from build123d import *

# Parameters (mm, degrees)
SKETCH2_R             = 14.49115295
CUT_EXTRUDE1_DEPTH    = 51.306406252
SKETCH3_R             = 5
EXTRUDE1_DEPTH        = 10
SKETCH5_R             = 9.901602584
SKETCH5_R_2           = 7
CUT_EXTRUDE2_DEPTH    = 3
IZIM2_R               = 4
KES_EKSTR_ZYON1_DEPTH = 220
IZIM3_R               = 4
KES_EKSTR_ZYON2_DEPTH = 40


with BuildPart() as part:
    # Sketch1 → Revolve1 (revolve)
    with BuildSketch(Plane.XY, mode=Mode.PRIVATE) as revolve1_sk:
        with BuildLine():
            Line((180.080433705, 44.141017842), (173.530538009, 44.141017842))
            ThreePointArc((173.530538009, 44.141017842), (172.538729892, 41.151971535), (173.530538009, 38.162925228))
            Line((173.530538009, 38.162925228), (180.080433705, 38.162925228))
            Line((180.080433705, 38.162925228), (180.080433705, 44.141017842))
        make_face()
        with BuildLine():
            Line((186.630329401, 44.141017842), (180.080433705, 44.141017842))
            Line((180.080433705, 44.141017842), (180.080433705, 38.162925228))
            Line((180.080433705, 38.162925228), (186.630329401, 38.162925228))
            ThreePointArc((186.630329401, 38.162925228), (187.103282451, 38.934012994), (187.429565668, 39.777695512))
            ThreePointArc((187.429565668, 39.777695512), (187.540311425, 42.052840793), (186.630329401, 44.141017842))
        make_face()
        with BuildLine():
            Line((180.080433705, 38.162925228), (180.080433705, 32.650327481))
            Line((180.080433705, 32.650327481), (187.735613173, 32.650327481))
            ThreePointArc((187.735613173, 32.650327481), (187.427007794, 35.455556025), (186.630329401, 38.162925228))
            Line((186.630329401, 38.162925228), (180.080433705, 38.162925228))
        make_face()
        with BuildLine():
            ThreePointArc((173.530538009, 38.162925228), (172.733859616, 35.455556025), (172.425254237, 32.650327481))
            Line((172.425254237, 32.650327481), (180.080433705, 32.650327481))
            Line((180.080433705, 32.650327481), (180.080433705, 38.162925228))
            Line((180.080433705, 38.162925228), (173.530538009, 38.162925228))
        make_face()
        with BuildLine():
            Line((173.530538009, 44.141017842), (169.927279386, 39.777695512))
            Line((169.927279386, 39.777695512), (169.927279386, 32.650327481))
            Line((169.927279386, 32.650327481), (172.425254237, 32.650327481))
            ThreePointArc((172.425254237, 32.650327481), (172.733859616, 35.455556025), (173.530538009, 38.162925228))
            ThreePointArc((173.530538009, 38.162925228), (172.538729892, 41.151971535), (173.530538009, 44.141017842))
        make_face()
        with BuildLine():
            ThreePointArc((186.630329401, 38.162925228), (187.427007794, 35.455556025), (187.735613173, 32.650327481))
            Line((187.735613173, 32.650327481), (189.375361044, 32.650327481))
            Line((189.375361044, 32.650327481), (189.375361044, 39.777695512))
            Line((189.375361044, 39.777695512), (187.429565668, 39.777695512))
            ThreePointArc((187.429565668, 39.777695512), (187.103282451, 38.934012994), (186.630329401, 38.162925228))
        make_face()
        Polygon((189.375361044, 39.777695512), (189.375361044, 32.650327481), (191.146824361, 32.650327481), (191.146824361, 42.553378699), (189.375361044, 42.553378699), align=None)
    revolve(revolve1_sk.sketch.rotate(Axis((-32.579678715, 32.650327481, 0), (1, 0, 0)), 90), axis=Axis((-32.579678715, 32.650327481, 0), (1, 0, 0)))

    # Sketch2 → Cut-Extrude1 (cut, through all)
    with BuildSketch(Plane.ZY.offset(-169.927279386)):
        with Locations((0, 32.650327481)):
            Circle(SKETCH2_R)
        Polygon((0, 44.141017842), (-9.95122976, 38.395672661), (-9.95122976, 26.9049823), (0, 21.15963712), (9.95122976, 26.9049823), (9.95122976, 38.395672661), align=None, mode=Mode.SUBTRACT)
    extrude(amount=-CUT_EXTRUDE1_DEPTH, mode=Mode.SUBTRACT)

    # Sweep3: sweep along a curve in space
    with BuildLine() as sweep3_path:
        Line((-222.210887695, 24.006507797, -16.672116117), (-222.346014244, 12.594218126, 18.492799117))
        ThreePointArc((-202.211021283, 30.157684617, -35.625859644), (-216.32728873, 28.357408148, -30.07863194), (-222.210887695, 24.006507797, -16.672116117))
        Line((-177.748857503, 30.157684617, -35.625859644), (-202.211021283, 30.157684617, -35.625859644))
        ThreePointArc((-157.748857503, 41.483617341, -19.141829556), (-163.606721879, 33.474973508, -30.797799013), (-177.748857503, 30.157684617, -35.625859644))
        Line((-157.748857503, 48.387877179, -9.093206659), (-157.748857503, 41.483617341, -19.141829556))
        ThreePointArc((-146.882458064, 52.727054495, 0), (-154.498514664, 52.19594197, -2.719947791), (-157.748857503, 48.387877179, -9.093206659))
        Line((-33.438092351, 32.801103659, 0), (-146.882458064, 52.727054495, 0))
        ThreePointArc((-31.708124112, 32.650327481, 0), (-32.576387258, 32.688092836, 0), (-33.438092351, 32.801103659, 0))
        Line((-31.708124112, 32.650327481, 0), (169.927279386, 32.650327481, 0))
    # Sketch3 → Sweep3 (sweep)
    with BuildSketch(Plane.ZY.offset(-169.927279386)):
        with Locations((0, 32.650327481)):
            Circle(SKETCH3_R)
    sweep(path=sweep3_path.line)

    # Sketch4 → Extrude1 (add)
    with BuildSketch(Plane(origin=(-0.053050316, -4.480433927, 13.805650207), x_dir=(0.9999933205859823, -0.0011282410835596105, 0.0034764716996236633), z_dir=(-0.003654966952096285, -0.30868502023615024, 0.9511572948247765))):
        Polygon((-226.140355235, 24.796964016), (-230.374247953, 17.911654597), (-226.528341443, 10.802341238), (-218.448542214, 10.578337297), (-214.214649497, 17.463646715), (-218.060556007, 24.572960075), align=None)
    extrude(amount=-EXTRUDE1_DEPTH)

    # Sketch5 → Cut-Extrude2 (cut)
    with BuildSketch(Plane(origin=(-0.053050316, -4.480433927, 13.805650207), x_dir=(0.9999933205859823, -0.0011282410835596105, 0.0034764716996236633), z_dir=(-0.003654966952096285, -0.30868502023615024, 0.9511572948247765))):
        with Locations((-222.294448725, 17.687650656)):
            Circle(SKETCH5_R)
        with Locations(Location((-222.294448725, 17.687650656, 0), (0, 0, 270))):
            Circle(SKETCH5_R_2, mode=Mode.SUBTRACT)
    extrude(amount=-CUT_EXTRUDE2_DEPTH, mode=Mode.SUBTRACT)

    # Çizim2 → Kes-Ekstrüzyon1 (cut)
    with BuildSketch(Plane(origin=(191.146824361, 0, 0), x_dir=(0, 0, -1), z_dir=(1, 0, 0))):
        with Locations((0, 32.650327481)):
            Circle(IZIM2_R)
    extrude(amount=-KES_EKSTR_ZYON1_DEPTH, mode=Mode.SUBTRACT)

    # Çizim3 → Kes-Ekstrüzyon2 (cut)
    with BuildSketch(Plane(origin=(-0.053050316, -4.480433927, 13.805650207), x_dir=(0.9999933205859823, -0.0011282410835595914, 0.003476471699623597), z_dir=(-0.003654966952096216, -0.3086850202361507, 0.9511572948247764))):
        with Locations(Location((-222.294448725, 17.687650656, 0), (0, 0, 270))):
            Circle(IZIM3_R)
    extrude(amount=-KES_EKSTR_ZYON2_DEPTH, mode=Mode.SUBTRACT)


solid = part.part
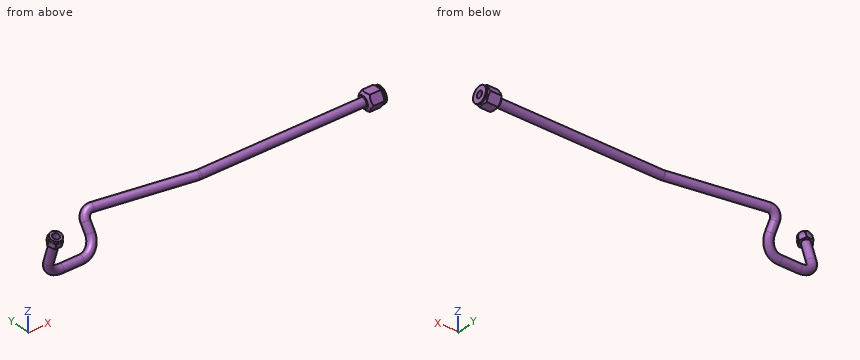
Can you work these out from the model? Positions are in its coordinate system, mm. Coordinates: 2 decimals unless noted, no trailing zeros. Order: outer loops, then holes, each group sorted by start corner. A loop starts at its lowest first (then second) coordinate and runs counter-clockwise, first axis right, second up. Notation, with made-up numbers: (-10, 80) - (28, 80) arc R14 cw to (28, 101) - close; hole circle Ø6 at (70.5, -10). An arc over 180 degrees is marked (long way). Answer as a JSON object with one key per item and string values. Group by question number.
Q1. Imagine slicing it at B-B (x = -189). Please give me the cut outline in (y, z), and give its area (3 significant figures).
Q2. Imagine slicing it at A-A (x = 164.5). Please give me the cut outline in (y, z), and give its area (3 significant figures).
Q3. Will these pins go through, and if not, where does the flat tip stop? P1, Ø5.5, axis at x = 183, y = 32.5, coming from the +Z side; P2, Ø3.5, axis at x = 177.5, y = 35, coming from the -Z side; P3, Ø1.5, axis at x = -43, z = -3, coming from the -Y side.
Q4. I need wall thicknesses on line 1 (Y direction, x = 67, z = 0); line 2 (X direction, y = 33.5, z = 9.5); line 3 (Z direction, x = -75.5, y = 42.5). Which ranges of each line are inside material? Lowest first, please. Write a range as from..to.
Determined:
{
 "1": {"outline": "circle Ø10 at (30.16, -35.63)", "area": "78.5 mm2"},
 "2": {"outline": "circle Ø10 at (32.65, 0); hole circle Ø8 at (32.65, 0)", "area": "28.3 mm2"},
 "3": {"P1": "stops at z = 9.95", "P2": "stops at z = -9.95", "P3": "stops at y = 29.93"},
 "4": {"line 1": "y = 27.65..28.65, 36.65..37.65", "line 2": "x = 171.92..187.51, 189.38..191.15", "line 3": "z = -4.45..4.45"}
}
